Autodesk Inventor part; units mm, degrees
ref_plane "XZ Plane" through (0, 0, 0) normal (0, 1, 0) x (-1, 0, 0)
ref_plane "XY Plane" through (0, 0, 0) normal (0, 0, 1) x (1, 0, 0)
sketch "Sketch1" plane through (0, 0, 0) normal (0, 1, 0) x (-1, 0, 0)
  circle A0 centre (0, 0) radius 12.7
  circle A1 centre (0, 0) radius 15.875
  dimension "d0" = 25.4
  dimension "d1" = 3.175
extrude "Extrusion1" add sketch "Sketch1" along normal blind 76.2
ref_plane "Work Plane1" through (15.875, 0, 0) normal (1, 0, 0) x (0, 1, 0)
sketch "Sketch2" plane through (15.875, 0, 0) normal (1, 0, 0) x (0, 1, 0)
  line L0 (63.5, 12.7) -> (38.1, 12.7)
  line L1 (38.1, 12.7) -> (38.1, -12.7)
  line L2 (38.1, -12.7) -> (63.5, -12.7)
  line L3 (63.5, -12.7) -> (63.5, 12.7)
  line L4 (76.2, -15.875) -> (76.2, 15.875)
  line L5 (72.39, 6.35) -> (66.04, 6.35)
  line L6 (66.04, 6.35) -> (66.04, -6.35)
  line L7 (66.04, -6.35) -> (72.39, -6.35)
  line L8 (72.39, -6.35) -> (72.39, 6.35)
  point P0 (0, 0)
  point P1 (63.5, 0)
  point P2 (66.04, 0)
  dimension "d4" = 25.4
  dimension "d5" = 25.4
  dimension "d6" = 12.7
  dimension "d7" = 2.54
  dimension "d8" = 6.35
  dimension "d13" = 12.7
extrude "Extrusion2" cut sketch "Sketch2" against normal up to next contours L3 L2 L1 L0
extrude "Extrusion3" add sketch "Sketch2" along normal blind 12.7 contours L8 L7 L6 L5
sketch "Sketch3" plane through (15.875, 72.39, 0) normal (0, 1, 0) x (1, 0, 0)
  point P0 (-15.875, 0)
extrude "Extrusion4" add sketch "Sketch2" against normal up to next contours L8 L7 L6 L5
sketch "Sketch4" plane through (14.5497, 72.39, 6.35) normal (0, 1, 0) x (1, 0, 0)
  line L0 (0, 12.7) -> (14.0253, 12.7)
  line L1 (14.0253, 12.7) -> (14.0253, 0)
  point P0 (-14.5497, 6.35)
  point P1 (7.0127, 6.35)
  point P2 (7.0127, 12.7)
  point P3 (14.0253, 6.35)
hole "Hole1" at (21.5623, 72.39, 0) direction (0, -1, 0) diameter 6.35 end up to surface
properties part number "MainBody"
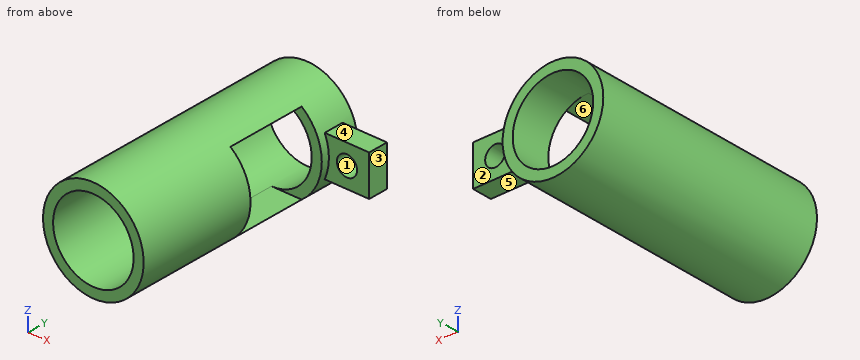
Could you check a few things on this model? Use its own coordinates, in mm. Face numbers are marked on the shaded views. A direction names the side the tool comes from. Round coordinates to 2 decimals unless told otherwise and drop trailing zeros. Write each loop counter-clockwise with the first axis right and the second up, starting at its lowest first coordinate (ties: lowest second). Pieces come first, ordered by that corner, then holes. Notation, with made-up numbers: (14.5, 12) - (27.5, 12) arc R21 cw to (27.5, 42) - close; hole circle Ø4 at (76.25, 58). An arc over 180 degrees is marked (long way). Use a Markdown table: item, result.
Q1. Please list where these lines run through material, in increasing order: L1, parallel to X at y = 71.25, z = 0 (3 decimals); L2, parallel to Z at x = -0.5, y = 17; L3, parallel to Y at x = 10.5, z = -8.
Output values:
| item | result |
|---|---|
| L1 | -15.875 to -12.7, 12.7 to 18.387, 24.737 to 28.575 |
| L2 | -15.87 to -12.69, 12.69 to 15.87 |
| L3 | 0 to 38.1, 63.5 to 76.2 |
Q2. I want a section at C-C (z = 0). List the corners of the cut face in (x, y) for me (3 decimals).
Output values:
| item | result |
|---|---|
| outline | (-15.875, 0) - (-12.7, 0) - (-12.7, 76.2) - (-15.875, 76.2) - close; (12.7, 0) - (15.875, 0) - (15.875, 38.1) - (12.7, 38.1) - close; (12.7, 63.5) - (15.875, 63.5) - (15.875, 66.04) - (18.387, 66.04) - (18.387, 72.39) - (15.875, 72.39) - (15.875, 76.2) - (12.7, 76.2) - close; (24.737, 66.04) - (28.575, 66.04) - (28.575, 72.39) - (24.737, 72.39) - close |
Q3. Thinking about a two-plate mould opening in X: for the marked faces 1, 2 and 3, which applies, released by +X, released by -X, zero draft, split by the parting line, or undercut?
Output values:
| item | result |
|---|---|
| face 1 | undercut |
| face 2 | zero draft |
| face 3 | released by +X |
Q4. I want a section at A-A (z = -4). List the corners of the cut face in (x, y) for me (3 decimals).
Output values:
| item | result |
|---|---|
| outline | (-15.363, 0) - (-12.054, 0) - (-12.054, 76.2) - (-15.363, 76.2) - close; (12.054, 0) - (15.363, 0) - (15.363, 38.1) - (12.054, 38.1) - close; (12.054, 63.5) - (15.363, 63.5) - (15.363, 66.04) - (28.575, 66.04) - (28.575, 72.39) - (15.363, 72.39) - (15.363, 76.2) - (12.054, 76.2) - close |
Q5. For the marked faces 4, 5 and 6, which set-ups out of +Z, -Z, +X, -X, +Y, -Y let a thin tool reach every point of the face, with its end or its side?
Output values:
| item | result |
|---|---|
| face 4 | +Z, +X, +Y, -Y |
| face 5 | -Z, +X, +Y, -Y |
| face 6 | +X |
Q6. I want a section at D-D (y = 22.5). List the corners of the cut face in (x, z) for me (3 decimals), plus the area to 3 significant figures.
Output values:
| item | result |
|---|---|
| outline | circle Ø31.75 at (0, 0); hole circle Ø25.4 at (0, 0) |
| area | 285 mm2 |
Q7. I want a section at B-B (x = 1.5). List the corners of the cut face in (y, z) for me, plus the area to 3 significant figures.
Output values:
| item | result |
|---|---|
| outline | (0, -15.8) - (76.2, -15.8) - (76.2, -12.61) - (63.5, -12.61) - (63.5, -12.7) - (38.1, -12.7) - (38.1, -12.61) - (0, -12.61) - close; (0, 12.61) - (38.1, 12.61) - (38.1, 12.7) - (63.5, 12.7) - (63.5, 12.61) - (76.2, 12.61) - (76.2, 15.8) - (0, 15.8) - close |
| area | 482 mm2 |
Q8. For pin 1 (8 mm diameter, centred on x = -10, z = 1, fed in from -Y); pin 2 (10 mm diameter, centred on x = 23, z = 3, fed in from -Y); pin 3 (2 mm diameter, centred on x = 9, y = 64, fed in from +Z); pin 4 (10 mm diameter, centred on x = -6.5, z = -1.5, fed in from +Y), each with a flat end and sliding along its axis, tell me the tip position at first contact or that it passes through.
Output values:
| item | result |
|---|---|
| pin 1 | y = 0 |
| pin 2 | y = 66.04 |
| pin 3 | z = 13.71 |
| pin 4 | through |
